from build123d import *

# Parameters (mm, degrees)
F1_DEPTH       = 130
F2_R           = 8
F4_D           = 6
F4_CSINK_D     = 8
F4_CSINK_ANGLE = 90
F6_D           = 6
F6_CSINK_D     = 8
F6_CSINK_ANGLE = 90


with BuildPart() as f1:
    # F0 (on Top) → F1 (new body)
    with BuildSketch(Plane.XY):
        with BuildLine():
            Line((20, -3), (20, 0))
            Line((20, 0), (5, 0))
            ThreePointArc((5, 0), (1.4644660941, -1.4644660941), (0, -5))
            Line((0, -5), (0, -20))
            Line((0, -20), (3, -20))
            Line((3, -20), (3, -6))
            ThreePointArc((3, -6), (3.8786796564, -3.8786796564), (6, -3))
            Line((6, -3), (20, -3))
        make_face()
    extrude(amount=F1_DEPTH)

    # F2
    f2_edges = [f1.edges().sort_by_distance(p)[0] for p in [
        (20, -1.5, 130),
        (20, -1.5, 0),
        (1.5, -20, 0),
        (1.5, -20, 130),
    ]]
    fillet(f2_edges, radius=F2_R)

    # F4 (through all)
    with Locations(Plane.XZ.offset(3)):
        with Locations((12, 122), (12, 65), (12, 8)):
            CounterSinkHole(F4_D / 2, F4_CSINK_D / 2, counter_sink_angle=F4_CSINK_ANGLE)

    # F6 (through all)
    with Locations(Plane.YZ.offset(3)):
        with Locations((-12, 122), (-12, 65), (-12, 8)):
            CounterSinkHole(F6_D / 2, F6_CSINK_D / 2, counter_sink_angle=F6_CSINK_ANGLE)


solid = f1.part
Verification items for the finished model (mm, model axes). A direction names the side the tool comes from. Round coordinates to 2 decimals unless told otherwise and drop trailing zeros. Loops run counter-clockwise (first coordinate to the right, second up) from the corner with the lowest first, then second, coordinate; pieces in that order, holes last. Notation, with made-up numbers: (11.25, 56.5) - (68.25, 56.5) arc R3 ccw to (68.25, 60.5) - close; hole circle Ø9 at (16.5, -5.75). An arc over 180 degrees is marked (long way). Use a Markdown table: item, result. Add a question column.
1. Section check D-D, the plane x = 17.5. Record the boundary of the cut face in (y, z).
2. Gauge pin test, flat ends, axial feed: pin 1 (1.5 mm diameter, centred on x = 3, z = 58, fed in from +Y); pin 2 (2 mm diameter, centred on x = 13, z = 110.5, fed in from -Y); pin 3 (7 mm diameter, centred on y = -12, z = 48.5, fed in from +X). Record the tip position at first contact, or that the pin passes through.
3. Release check for a two-part mould opening along Y. For faces 1 (the face through (1, -12, 125)), 2 (the face through (17.719, -1.479, 127.594)), 3 (the face through (2, -1, 64)), 4 (the face through (1.521, -17.719, 2.406)) record: released by +Y, released by -Y, zero draft, split by the parting line, or undercut.
4. Section check A-A, the plane z = 65. Record the boundary of the cut face in (x, y).
5. Thickness scan on probe 1 along Z at (x, y) = (0.55, -12); probe 2 along Y at (x, z) = (1, 8); probe 3 along Y at (x, z) = (14.5, 118.5). Record the ranges inside material, lowest first. Write a range as [from, to].
6. Access from +Z, -Z, +X, -X, +Y, -Y to the whole of each face (thin tool, end or side, straight path). Record for faces 5 (the face through (3, -16.2, 64.1)), 6 (the face through (12, -1, 125)).
7. Section check C-C, the plane y = -13.75. Give the number of separate pieces and of enclosed holes in the cut face, plus the area to 3 significant figures.
8. Section check B-B, the plane z = 93. Record the boundary of the cut face in (x, y).
Checks:
| question | item | result |
|---|---|---|
| 1 | outline | (-3, 2.19) - (0, 2.19) - (0, 127.81) - (-3, 127.81) - close |
| 2 | pin 1 | stops at y = -0.16 |
| 2 | pin 2 | stops at y = -3 |
| 2 | pin 3 | stops at x = 3 |
| 3 | face 1 | undercut |
| 3 | face 2 | zero draft |
| 3 | face 3 | released by +Y |
| 3 | face 4 | released by -Y |
| 4 | outline | (0, -20) - (3, -20) - (3, -16) - (2, -15) - (0, -15) - close; (0, -9) - (2, -9) - (3, -8) - (3, -6) arc R3 cw to (6, -3) - (8, -3) - (9, -2) - (9, 0) - (5, 0) arc R5 ccw to (0, -5) - close; (15, -2) - (16, -3) - (20, -3) - (20, 0) - (15, 0) - close |
| 5 | probe 1 | z = [0, 5], [11, 62], [68, 119], [125, 130] |
| 5 | probe 2 | y = [-20, -15], [-9, -2] |
| 5 | probe 3 | y = [-3, 0] |
| 6 | face 5 | +Z, -Z, +X, -Y |
| 6 | face 6 | +Y, -Y |
| 7 | separate pieces | 4 |
| 7 | enclosed holes | 0 |
| 7 | area | 341 mm^2 |
| 8 | outline | (0, -20) - (3, -20) - (3, -6) arc R3 cw to (6, -3) - (20, -3) - (20, 0) - (5, 0) arc R5 ccw to (0, -5) - close |
